Can you work these out from the model? Positions are in its coordinate system, mm. Give positions to 0.01 mm unless a question says otherwise; leave off trailing zeros. Loops run counter-clockwise (first coordinate to the right, second up) from the corner with the lowest first, then second, coordinate; pieces in that order, holes last. Notation, with made-up numbers: (56, -31.5) - (98, -31.5) arc R14 ccw to (98, -11.5) - close; hole circle Ø6 at (2, -23.5). An arc over 180 degrees is marked (long way). Answer as a JSON object with one key per item and string values.
```python
from build123d import *

# Parameters (mm, degrees)
SKETCH_1_W                   = 40
SKETCH_1_H                   = 80
SM_BASE_FLANGE_1_DEPTH       = 3
OTHER_START                  = -3
OTHER_1_DEPTH                = 3
HOLE_WIZARD_M8_1_D           = 9
HOLE_WIZARD_M8_1_DEPTH       = 12.4
HOLE_WIZARD_M8_1_CSINK_D     = 9.05
HOLE_WIZARD_M8_1_CSINK_ANGLE = 90
HOLE_WIZARD_M8_1_TIP         = 2.703872786


# Read off the part's stored shape, not the designer's step: 断开-边角1
# Sheet-metal steps are written as plain solids
with BuildPart() as part:
    # Sketch 1 → 基体-法兰1 (new body)
    with BuildSketch(Plane.XY):
        Rectangle(SKETCH_1_W, SKETCH_1_H)
    extrude(amount=-SM_BASE_FLANGE_1_DEPTH)

    # Other 1 outline → Other 1 (cut)
    with BuildSketch(Plane.XY.offset(OTHER_START)):
        with BuildLine():
            ThreePointArc((20, -37), (19.121320344, -39.121320344), (17, -40))
            Line((17, -40), (20, -40))
            Line((20, -40), (20, -37))
        make_face()
        with BuildLine():
            Line((-20, -40), (-17, -40))
            ThreePointArc((-17, -40), (-19.121320344, -39.121320344), (-20, -37))
            Line((-20, -37), (-20, -40))
        make_face()
        with BuildLine():
            ThreePointArc((17, 40), (19.121320344, 39.121320344), (20, 37))
            Line((20, 37), (20, 40))
            Line((20, 40), (17, 40))
        make_face()
        with BuildLine():
            Line((-20, 40), (-20, 37))
            ThreePointArc((-20, 37), (-19.121320344, 39.121320344), (-17, 40))
            Line((-17, 40), (-20, 40))
        make_face()
    extrude(amount=OTHER_1_DEPTH, mode=Mode.SUBTRACT)

    # M8 间隙孔1
    with Locations(Plane.XY):
        with Locations((0, 20), (0, -20)):
            CounterSinkHole(HOLE_WIZARD_M8_1_D / 2, HOLE_WIZARD_M8_1_CSINK_D / 2, depth=HOLE_WIZARD_M8_1_DEPTH, counter_sink_angle=HOLE_WIZARD_M8_1_CSINK_ANGLE)
            with Locations((0, 0, -(HOLE_WIZARD_M8_1_DEPTH + HOLE_WIZARD_M8_1_TIP / 2))):  # 118° drill point
                Cone(0, HOLE_WIZARD_M8_1_D / 2, HOLE_WIZARD_M8_1_TIP, mode=Mode.SUBTRACT)


solid = part.part
```
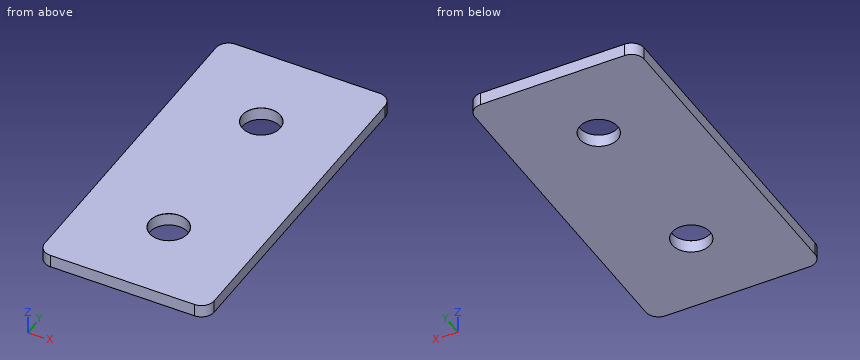
1) Imagine slicing it at B-B on x = 0. Write out the boundary of the cut face in (y, z) (3 decimals).
Check sheet entries:
{"outline": "(-40, -3) - (-24.5, -3) - (-24.5, -0.025) - (-24.525, 0) - (-40, 0) - close; (-15.5, -3) - (15.5, -3) - (15.5, -0.025) - (15.475, 0) - (-15.475, 0) - (-15.5, -0.025) - close; (24.5, -3) - (40, -3) - (40, 0) - (24.525, 0) - (24.5, -0.025) - close"}
2) I'm going to push a flat-ended pin straight in: P1, Ø7, axis at x = 0, y = 20, coming from the -Z side. Where does the tip first touch, or does it pass through?
Check sheet entries:
{"P1": "through"}
3) Imagine slicing it at A-A on y = -20. Write out the boundary of the cut face in (x, z) (3 decimals), and give its area (3 significant figures).
Check sheet entries:
{"outline": "(-20, -3) - (-4.5, -3) - (-4.5, -0.025) - (-4.525, 0) - (-20, 0) - close; (4.5, -3) - (20, -3) - (20, 0) - (4.525, 0) - (4.5, -0.025) - close", "area": "93.0 mm2"}
4) I need wall thicknesses on L1, parallel to Y at x = 0, z = -2.3; L2, parallel to X at y = 20, z = -0.6; L3, parallel to Y at x = 3, z = -0.7. Which ranges of each line are inside material? Lowest first, please.
Check sheet entries:
{"L1": "-40 to -24.5, -15.5 to 15.5, 24.5 to 40", "L2": "-20 to -4.5, 4.5 to 20", "L3": "-40 to -23.35, -16.65 to 16.65, 23.35 to 40"}
5) Imagine slicing it at C-C on z = -2.15. Write out the boundary of the cut face in (x, y).
Check sheet entries:
{"outline": "(-20, -37) arc R3 ccw to (-17, -40) - (17, -40) arc R3 ccw to (20, -37) - (20, 37) arc R3 ccw to (17, 40) - (-17, 40) arc R3 ccw to (-20, 37) - close; hole circle Ø9 at (0, -20); hole circle Ø9 at (0, 20)"}
